Build history of the part. All positions in model axes, mm. Face numbers are marked on the shaded views. A direction names the side the tool comes from. Round coordinates to 2 decimals unless told otherwise and drop trailing zeros. Loops run counter-clockwise (first coordinate to the right, second up) from the corner with the lowest first, then second, coordinate; pieces in that order, holes last.
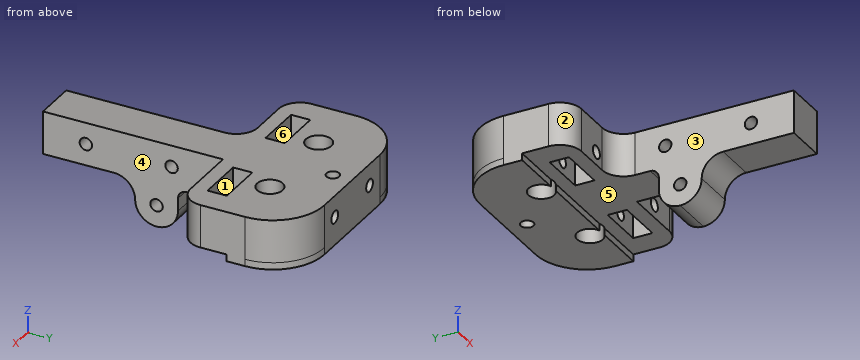
from build123d import *

# Parameters (mm, degrees)
SKETCH1_W               = 48
SKETCH1_H               = 70
BOSS_EXTRUDE1_DEPTH     = 10
SKETCH2_R               = 3
CUT_EXTRUDE1_DEPTH      = 86.463442477
SKETCH3_W               = 20.6
SKETCH3_H               = 20.6
CUT_EXTRUDE2_DEPTH      = 86.463442477
FILLET1_R               = 12
SKETCH4_R               = 1.5
CUT_EXTRUDE3_DEPTH      = 86.463442477
SKETCH5_R               = 1.45
CUT_EXTRUDE4_DEPTH      = 10
CUT_EXTRUDE5_DEPTH      = 86.463442477
CUT_EXTRUDE5_DEPTH_BACK = 86.463442477
SKETCH7_W               = 11
SKETCH7_H               = 4.5
SKETCH11_W              = 32
SKETCH11_H              = 15
CUT_EXTRUDE6_DEPTH      = 86.463442477
CUT_EXTRUDE7_DEPTH      = 8
CUT_EXTRUDE7_DEPTH_BACK = 5
SKETCH12_R              = 1.5
SKETCH13_R              = 1.5
BOSS_EXTRUDE4_DEPTH     = 1.6
FILLET2_R               = 8
SKETCH14_W              = 48
SKETCH14_H              = 42.571441548
CUT_EXTRUDE8_DEPTH      = 86.665395594
SKETCH15_W              = 10
SKETCH15_H              = 10
BOSS_EXTRUDE5_DEPTH     = 42
SKETCH18_W              = 10
SKETCH18_H              = 10
BOSS_EXTRUDE8_DEPTH     = 10
SKETCH19_R              = 1.45
CUT_EXTRUDE9_DEPTH      = 76.903390772
FILLET3_R               = 5
FILLET4_R               = 5
FILLET5_R               = 2


# Some blends are built 0.0001 mm under size
with BuildPart() as part:
    # Sketch1 → Boss-Extrude1 (new body)
    with BuildSketch(Plane.XY):
        with Locations((24, -35)):
            Rectangle(SKETCH1_W, SKETCH1_H)
    extrude(amount=BOSS_EXTRUDE1_DEPTH)

    # Sketch2 → Cut-Extrude1 (cut, through all)
    with BuildSketch(Plane.XY.offset(10)):
        with Locations((13.5, -13.5)):
            Circle(SKETCH2_R)
        with Locations((34.5, -13.5)):
            Circle(SKETCH2_R)
    extrude(amount=-CUT_EXTRUDE1_DEPTH, mode=Mode.SUBTRACT)

    # Sketch3 → Cut-Extrude2 (cut, through all)
    with BuildSketch(Plane.XY.offset(10)):
        with Locations((24, -48.8)):
            Rectangle(SKETCH3_W, SKETCH3_H)
    extrude(amount=-CUT_EXTRUDE2_DEPTH, mode=Mode.SUBTRACT)

    # Fillet1
    fillet1_edges = [part.edges().sort_by_distance(p)[0] for p in [
        (0, 0, 5),
        (48, 0, 5),
    ]]
    fillet(fillet1_edges, radius=FILLET1_R)

    # Sketch4 → Cut-Extrude3 (cut, through all)
    with BuildSketch(Plane(origin=(0, 0, 0), x_dir=(-1, 0, 0), z_dir=(0, 0, -1))):
        with Locations((-24, -4.5)):
            Circle(SKETCH4_R)
    extrude(amount=-CUT_EXTRUDE3_DEPTH, mode=Mode.SUBTRACT)

    # Sketch5 → Cut-Extrude4 (cut)
    with BuildSketch(Plane(origin=(0, 0, 0), x_dir=(1, 0, 0), z_dir=(0, 1, 0))):
        with Locations(Location((16.5, -5, 0), (0, 0, 270))):
            Circle(SKETCH5_R)
        with Locations(Location((31.5, -5, 0), (0, 0, 270))):
            Circle(SKETCH5_R)
    extrude(amount=-CUT_EXTRUDE4_DEPTH, mode=Mode.SUBTRACT)

    # Sketch7 → Cut-Extrude5 (cut, two sides: drawn at the far end of the back side and taken through both)
    with BuildSketch(Plane(origin=(0, 0, 0), x_dir=(-1, 0, 0), z_dir=(0, 0, -1)).offset(-CUT_EXTRUDE5_DEPTH_BACK)):
        with Locations((-36.5, -21.75)):
            Rectangle(SKETCH7_W, SKETCH7_H)
        with Locations((-11.5, -21.75)):
            Rectangle(SKETCH7_W, SKETCH7_H)
    extrude(amount=CUT_EXTRUDE5_DEPTH + CUT_EXTRUDE5_DEPTH_BACK, mode=Mode.SUBTRACT)

    # Sketch11 → Cut-Extrude6 (cut, through all)
    with BuildSketch(Plane(origin=(0, 0, 0), x_dir=(-1, 0, 0), z_dir=(0, 0, -1))):
        with Locations((-24, -35)):
            Rectangle(SKETCH11_W, SKETCH11_H)
    extrude(amount=-CUT_EXTRUDE6_DEPTH, mode=Mode.SUBTRACT)

    # Sketch12 → Cut-Extrude7 (cut, two sides: drawn at the far end of the back side and taken through both)
    with BuildSketch(Plane(origin=(0, -24, 0), x_dir=(1, 0, 0), z_dir=(0, 1, 0)).offset(-CUT_EXTRUDE7_DEPTH_BACK)):
        with Locations(Location((36.5, -3, 0), (0, 0, 90))):
            Circle(SKETCH12_R)
        with Locations((11.5, -3)):
            Circle(SKETCH12_R)
    extrude(amount=CUT_EXTRUDE7_DEPTH + CUT_EXTRUDE7_DEPTH_BACK, mode=Mode.SUBTRACT)

    # Sketch13 → Boss-Extrude4 (add)
    with BuildSketch(Plane(origin=(0, 0, 0), x_dir=(-1, 0, 0), z_dir=(0, 0, -1))):
        with BuildLine():
            Line((-48, -12), (-48, -16.3))
            Line((-48, -16.3), (-35.577032961, -16.3))
            ThreePointArc((-35.577032961, -16.3), (-36.198367027, -11.027036304), (-31.5, -13.5))
            ThreePointArc((-31.5, -13.5), (-32.027036304, -15.198367027), (-33.422967039, -16.3))
            Line((-33.422967039, -16.3), (-14.577032961, -16.3))
            ThreePointArc((-14.577032961, -16.3), (-15.198367027, -11.027036304), (-10.5, -13.5))
            ThreePointArc((-10.5, -13.5), (-11.027036304, -15.198367027), (-12.422967039, -16.3))
            Line((-12.422967039, -16.3), (0, -16.3))
            Line((0, -16.3), (0, -12))
            ThreePointArc((0, -12), (-3.514718626, -3.514718626), (-12, 0))
            Line((-12, 0), (-36, 0))
            ThreePointArc((-36, 0), (-44.485281374, -3.514718626), (-48, -12))
        make_face()
        with Locations((-24, -4.5)):
            Circle(SKETCH13_R, mode=Mode.SUBTRACT)
    extrude(amount=BOSS_EXTRUDE4_DEPTH)

    # Fillet2
    # the kernel refuses this fillet: 8 mm, written as the material it takes off along each edge
    with BuildSketch(Plane(origin=(13.7, -42.5, -19.155612754), x_dir=(-1, 0, 0), z_dir=(0, 0, 1))) as fillet2_piece_1:
        with BuildLine():
            CenterArc((8, 7.662245102), FILLET2_R, 180, 73.291656284)
            Line((0, 7.662245102), (-0.16, 7.662245102))
            Line((-0.16, 7.662245102), (-0.16, 0))
            Line((-0.16, 0), (0, -0.16))
            ThreePointArc((0, -0.16), (2.85, -0.16), (5.654, -0.153244902))
            Line((5.654, -0.153244902), (5.7, 0))
        make_face()
    extrude(amount=48.311225509, mode=Mode.SUBTRACT)
    with BuildSketch(Plane(origin=(34.3, -42.5, 29.155612754), x_dir=(0, -1, 0), z_dir=(0, 0, -1))) as fillet2_piece_2:
        with BuildLine():
            CenterArc((7.662245102, -8), FILLET2_R, 90, 73.291656284)
            Line((0, -5.7), (-0.153244902, -5.654))
            ThreePointArc((-0.153244902, -5.654), (-0.16, -2.85), (-0.16, 0))
            Line((-0.16, 0), (0, 0.16))
            Line((0, 0.16), (7.662245102, 0.16))
            Line((7.662245102, 0.16), (7.662245102, 0))
        make_face()
    extrude(amount=48.311225509, mode=Mode.SUBTRACT)

    # Sketch14 → Cut-Extrude8 (cut, through all)
    with BuildSketch(Plane.XY.offset(10)):
        with Locations((24, -48.714279226)):
            Rectangle(SKETCH14_W, SKETCH14_H)
    extrude(amount=-CUT_EXTRUDE8_DEPTH, mode=Mode.SUBTRACT)

    # Sketch15 → Boss-Extrude5 (add)
    with BuildSketch(Plane(origin=(0, -27.428558452, 0), x_dir=(-1, 0, 0), z_dir=(0, -1, 0))):
        with Locations((-24, -5)):
            Rectangle(SKETCH15_W, SKETCH15_H)
    extrude(amount=BOSS_EXTRUDE5_DEPTH)

    # Sketch18 → Boss-Extrude8 (add)
    with BuildSketch(Plane(origin=(0, 0, 0), x_dir=(-1, 0, 0), z_dir=(0, 0, -1))):
        with Locations((-24, -42.928558452)):
            Rectangle(SKETCH18_W, SKETCH18_H)
    extrude(amount=BOSS_EXTRUDE8_DEPTH)

    # Sketch19 → Cut-Extrude9 (cut, through all)
    with BuildSketch(Plane(origin=(29, 0, 0), x_dir=(0, 0, -1), z_dir=(1, 0, 0))):
        with Locations((5, -42.928558452)):
            Circle(SKETCH19_R)
        with Locations((-5, -59.428558452)):
            Circle(SKETCH19_R)
        with Locations((-5, -39.428558452)):
            Circle(SKETCH19_R)
    extrude(amount=-CUT_EXTRUDE9_DEPTH, mode=Mode.SUBTRACT)

    # Fillet3
    fillet3_edges = [part.edges().sort_by_distance(p)[0] for p in [
        (48, -27.428558452, 5),
        (0, -27.428558452, 5),
        (19, -27.428558452, 5),
    ]]
    fillet(fillet3_edges, radius=FILLET3_R)

    # Fillet4
    fillet4_edges = [part.edges().sort_by_distance(p)[0] for p in [
        (24, -47.928558452, 0),
        (24, -47.928558452, -10),
        (24, -37.928558452, -10),
    ]]
    fillet(fillet4_edges, radius=FILLET4_R - 0.0001)  # a hair under: the kernel refuses the full size

    # Fillet5
    fillet5_edges = [part.edges().sort_by_distance(p)[0] for p in [
        (24, -37.928558452, 0),
    ]]
    fillet(fillet5_edges, radius=FILLET5_R)


solid = part.part
(1) Slice it at C-C on z = -8. List the corners of the cut face in (x, y), plus the area to 3 significant figures.
Responses:
outline: (19, -46.93) - (29, -46.93) - (29, -38.93) - (19, -38.93) - close
area: 80.0 mm2
(2) Which spindle directions (+Z, -Z, +X, -X, +Y, -Y) get a long thin tool onto all of the face, cutting with end or side? Do the marked faces 4, 5 and 6. Say none if no direction does.
Responses:
face 4: +Z, -Z, +X, -Y
face 5: -Z, +X, -X
face 6: +Z, -Z
(3) Slice it at B-B on x = 21. Count the separate pieces of the cut face and the enclosed holes in it, plus the area to 3 significant figures.
Responses:
separate pieces: 1
enclosed holes: 3
area: 796 mm2
(4) Pull direction Y, two halves, no side cores. Call the marked faces 1, 2 and 3: +Y half, -Y half, draft (parallel to the pull), parting line (faces both ways), or undercut.
Responses:
face 1: undercut
face 2: -Y half
face 3: draft
(5) Slice it at D-D on y = -26. List the corners of the cut face in (x, z), plus the area to 3 significant figures.
Responses:
outline: (1.5, 0) - (46.5, 0) - (46.5, 10) - (1.5, 10) - close; hole circle Ø3 at (11.5, 3); hole circle Ø3 at (36.5, 3)
area: 436 mm2
(6) Slice it at A-A on y = -4.5. List the corners of the cut face in (x, z).
Responses:
outline: (2.63, -1.6) - (22.5, -1.6) - (22.5, 10) - (2.63, 10) - close; (25.5, -1.6) - (45.37, -1.6) - (45.37, 10) - (25.5, 10) - close; hole circle Ø2.9 at (16.5, 5); hole circle Ø2.9 at (31.5, 5)
(7) Pin check, flat tips, straight feed: P1, Ø2.5, axis at x = 26, z = -3, coming from the +Y side; P2, Ø3, axis at y = -49.5, z = 0.5, coming from the -X side; P3, Ø10, axis at y = -59, z = 6.5, coming from the +X side; P4, Ø8, axis at x = 34.5, y = -13.5, coming from the +Z side. Stop position of each tip, or through.
Responses:
P1: stops at y = -37.91
P2: stops at x = 19
P3: stops at x = 29
P4: stops at z = 10
(8) Probe line 1 (Y direction, x = 34.5, z = 3.25); line 2 (X direction, y = -17.15, z = 3); line 3 (Y direction, x = 11, z = 8). List the from-to ranges inside material, lowest first.
Responses:
line 1: y = -27.43 to -24, -19.5 to -16.5, -10.5 to 0
line 2: x = 0 to 10, 13 to 35, 38 to 48
line 3: y = -27.43 to -24, -19.5 to -15.16, -11.84 to -0.04
